from build123d import *

# Parameters (mm, degrees)
SKETCH_1_W          = 107
SKETCH_1_H          = 31
SKETCH_1_W_2        = 26
SKETCH_1_H_2        = 4
SKETCH_1_W_3        = 25
SKETCH_1_H_3        = 9
EXTRUDE_1_DEPTH     = 2
EXTRUDE_2_DEPTH     = 2
CUT_EXTRUDE_1_DEPTH = 117.228223767
SKETCH_5_W          = 15
SKETCH_5_H          = 2.5
EXTRUDE_3_DEPTH     = 2
CUT_EXTRUDE_2_DEPTH = 117.919844338
CUT_EXTRUDE_3_DEPTH = 117.919844338


with BuildPart() as part:
    # 草图1 → 凸台-拉伸1 (new body)
    with BuildSketch(Plane(origin=(0, 0, 0), x_dir=(0, 0, -1), z_dir=(1, 0, 0))):
        with Locations((53.5, 15.5)):
            Rectangle(SKETCH_1_W, SKETCH_1_H)
        with Locations((72, 16)):
            Rectangle(SKETCH_1_W_2, SKETCH_1_H_2, mode=Mode.SUBTRACT)
        with Locations((40.5, 18.5)):
            Rectangle(SKETCH_1_W_3, SKETCH_1_H_3, mode=Mode.SUBTRACT)
    extrude(amount=EXTRUDE_1_DEPTH)

    # 草图2 → 凸台-拉伸2 (add)
    with BuildSketch(Plane(origin=(2, 0, 0), x_dir=(0, 0, -1), z_dir=(1, 0, 0))):
        Polygon((0, 31), (-5, 31), (-5, 0), (0, 0), (0, 5), (-2.1, 5), (-2.1, 13), (0, 13), (0, 18), (-2.1, 18), (-2.1, 26), (0, 26), align=None)
        Polygon((107, 0), (107, 5), (109.1, 5), (109.1, 13), (107, 13), (107, 18), (109.1, 18), (109.1, 26), (107, 26), (107, 31), (112, 31), (112, 0), align=None)
    extrude(amount=-EXTRUDE_2_DEPTH)

    # 草图3 → 切除-拉伸1 (cut, through all)
    with BuildSketch(Plane(origin=(2, 0, 0), x_dir=(0, 0, -1), z_dir=(1, 0, 0))):
        with BuildLine():
            Line((-2.1, 24), (-2.1, 26))
            ThreePointArc((-2.1, 26), (-3.1, 25), (-2.1, 24))
        make_face()
        with BuildLine():
            Line((0, 24), (0, 26))
            ThreePointArc((0, 26), (1, 25), (0, 24))
        make_face()
        with BuildLine():
            Line((0, 20), (0, 18))
            ThreePointArc((0, 18), (1, 19), (0, 20))
        make_face()
        with BuildLine():
            Line((-2.1, 20), (-2.1, 18))
            ThreePointArc((-2.1, 18), (-3.1, 19), (-2.1, 20))
        make_face()
        with BuildLine():
            Line((-2.1, 11), (-2.1, 13))
            ThreePointArc((-2.1, 13), (-3.1, 12), (-2.1, 11))
        make_face()
        with BuildLine():
            Line((0, 11), (0, 13))
            ThreePointArc((0, 13), (1, 12), (0, 11))
        make_face()
        with BuildLine():
            Line((0, 7), (0, 5))
            ThreePointArc((0, 5), (1, 6), (0, 7))
        make_face()
        with BuildLine():
            Line((-2.1, 7), (-2.1, 5))
            ThreePointArc((-2.1, 5), (-3.1, 6), (-2.1, 7))
        make_face()
        with BuildLine():
            Line((109.1, 7), (109.1, 5))
            ThreePointArc((109.1, 5), (110.1, 6), (109.1, 7))
        make_face()
        with BuildLine():
            Line((107, 7), (107, 5))
            ThreePointArc((107, 5), (106, 6), (107, 7))
        make_face()
        with BuildLine():
            Line((107, 11), (107, 13))
            ThreePointArc((107, 13), (106, 12), (107, 11))
        make_face()
        with BuildLine():
            Line((109.1, 11), (109.1, 13))
            ThreePointArc((109.1, 13), (110.1, 12), (109.1, 11))
        make_face()
        with BuildLine():
            Line((109.1, 20), (109.1, 18))
            ThreePointArc((109.1, 18), (110.1, 19), (109.1, 20))
        make_face()
        with BuildLine():
            Line((107, 20), (107, 18))
            ThreePointArc((107, 18), (106, 19), (107, 20))
        make_face()
        with BuildLine():
            Line((107, 24), (107, 26))
            ThreePointArc((107, 26), (106, 25), (107, 24))
        make_face()
        with BuildLine():
            Line((109.1, 24), (109.1, 26))
            ThreePointArc((109.1, 26), (110.1, 25), (109.1, 24))
        make_face()
    extrude(amount=-CUT_EXTRUDE_1_DEPTH, mode=Mode.SUBTRACT)

    # 草图5 → 凸台-拉伸3 (add)
    with BuildSketch(Plane(origin=(2, 0, 0), x_dir=(0, 0, -1), z_dir=(1, 0, 0))):
        with Locations((17.5, 32.25)):
            Rectangle(SKETCH_5_W, SKETCH_5_H)
        with Locations((53.5, 32.25)):
            Rectangle(SKETCH_5_W, SKETCH_5_H)
        with Locations((89.5, 32.25)):
            Rectangle(SKETCH_5_W, SKETCH_5_H)
        with Locations((89.5, -1.25)):
            Rectangle(SKETCH_5_W, SKETCH_5_H)
        with Locations((53.5, -1.25)):
            Rectangle(SKETCH_5_W, SKETCH_5_H)
        with Locations((17.5, -1.25)):
            Rectangle(SKETCH_5_W, SKETCH_5_H)
    extrude(amount=-EXTRUDE_3_DEPTH)

    # 草图6 → 切除-拉伸2 (cut, through all)
    with BuildSketch(Plane(origin=(2, 0, 0), x_dir=(0, 0, -1), z_dir=(1, 0, 0))):
        with BuildLine():
            Line((10, 31), (8, 31))
            ThreePointArc((8, 31), (9, 30), (10, 31))
        make_face()
        with BuildLine():
            Line((25, 31), (27, 31))
            ThreePointArc((27, 31), (26, 30), (25, 31))
        make_face()
        with BuildLine():
            Line((46, 31), (44, 31))
            ThreePointArc((44, 31), (45, 30), (46, 31))
        make_face()
        with BuildLine():
            Line((61, 31), (63, 31))
            ThreePointArc((63, 31), (62, 30), (61, 31))
        make_face()
        with BuildLine():
            Line((82, 31), (80, 31))
            ThreePointArc((80, 31), (81, 30), (82, 31))
        make_face()
        with BuildLine():
            Line((97, 31), (99, 31))
            ThreePointArc((99, 31), (98, 30), (97, 31))
        make_face()
        with BuildLine():
            Line((97, 0), (99, 0))
            ThreePointArc((99, 0), (98, 1), (97, 0))
        make_face()
        with BuildLine():
            Line((82, 0), (80, 0))
            ThreePointArc((80, 0), (81, 1), (82, 0))
        make_face()
        with BuildLine():
            Line((61, 0), (63, 0))
            ThreePointArc((63, 0), (62, 1), (61, 0))
        make_face()
        with BuildLine():
            Line((46, 0), (44, 0))
            ThreePointArc((44, 0), (45, 1), (46, 0))
        make_face()
        with BuildLine():
            Line((25, 0), (27, 0))
            ThreePointArc((27, 0), (26, 1), (25, 0))
        make_face()
        with BuildLine():
            Line((10, 0), (8, 0))
            ThreePointArc((8, 0), (9, 1), (10, 0))
        make_face()
    extrude(amount=-CUT_EXTRUDE_2_DEPTH, mode=Mode.SUBTRACT)

    # 草图7 → 切除-拉伸3 (cut, through all)
    with BuildSketch(Plane(origin=(2, 0, 0), x_dir=(0, 0, -1), z_dir=(1, 0, 0))):
        with BuildLine():
            Line((6, 28), (22, 28))
            ThreePointArc((22, 28), (25, 25), (22, 22))
            Line((22, 22), (6, 22))
            ThreePointArc((6, 22), (3, 25), (6, 28))
        make_face()
        with BuildLine():
            Line((6, 10), (31, 10))
            ThreePointArc((31, 10), (34, 7), (31, 4))
            Line((31, 4), (6, 4))
            ThreePointArc((6, 4), (3, 7), (6, 10))
        make_face()
        with BuildLine():
            Line((6, 19), (22, 19))
            ThreePointArc((22, 19), (25, 16), (22, 13))
            Line((22, 13), (6, 13))
            ThreePointArc((6, 13), (3, 16), (6, 19))
        make_face()
        with BuildLine():
            Line((41, 10), (66, 10))
            ThreePointArc((66, 10), (69, 7), (66, 4))
            Line((66, 4), (41, 4))
            ThreePointArc((41, 4), (38, 7), (41, 10))
        make_face()
        with BuildLine():
            Line((76, 10), (101, 10))
            ThreePointArc((101, 10), (104, 7), (101, 4))
            Line((101, 4), (76, 4))
            ThreePointArc((76, 4), (73, 7), (76, 10))
        make_face()
        with BuildLine():
            Line((59, 28), (101, 28))
            ThreePointArc((101, 28), (104, 25), (101, 22))
            Line((101, 22), (59, 22))
            ThreePointArc((59, 22), (56, 25), (59, 28))
        make_face()
        with BuildLine():
            Line((91, 19), (101, 19))
            ThreePointArc((101, 19), (104, 16), (101, 13))
            Line((101, 13), (91, 13))
            ThreePointArc((91, 13), (88, 16), (91, 19))
        make_face()
    extrude(amount=-CUT_EXTRUDE_3_DEPTH, mode=Mode.SUBTRACT)


solid = part.part
Geometry check sheet. Reference: the model listing, model coordinates, mm. A direction names the side the tool comes from. Coordinates: 2 decimals unless noted, no trailing zeros. Order: outer loops, then holes, each group sorted by start corner. A loop starts at its lowest first (then second) coordinate and runs counter-clockwise, first axis right, second up. Notation, with made-up numbers: (18, -15) - (74, -15) arc R18 ccw to (74, 2) - close; hole circle Ø3 at (52.5, 36). An arc over 180 degrees is marked (long way). Answer in a Markdown table with one row per item. Add a question column.
1) Cross-section at D-D, the plane x = 1.2. State how many separate pieces and enclosed holes the cut face has, then the cut area to 3 significant figures.
2) Cross-section at B-B, the plane z = -9. Record the cut outline in (x, y), then the cut area to 3 significant figures.
3) Set-up check for faces 1 (the flat face through (1, 32, -25)), 2 (the flat face through (1, 31, -106)), 3 (the flat face through (1, 0, -71)), 4 (the cylindrical face through (1, 19, -106)): record each of +Z, -Z, +X, -X, +Y, -Y from which the full face is reachable in a straight line by a thin tool's end or side.
4) Cross-section at C-C, the plane z = -39. Record the cut outline in (x, y).
5) Release check for a two-part mould opening along Z. For faces 5 (the flat face through (1, 0, -35)), 6 (the flat face through (1, -2.5, -53)), 7 (the flat face through (1, 16, -112)) record: +Z half, -Z half, draft (parallel to the pull), parting line (faces both ways), or undercut.
6) Material ranges on line 1 along Y through (x, z) = (1.1, -45); line 2 along Y through (x, z) = (0.35, -76.5); line 3 along Y through (x, z) = (1.05, -17.5), recorded low to high. Write a range as [from, to].
7) Cross-section at A-A, the plane y = 25. Record the cut outline in (x, z).
8) Gauge pin test, flat ends, axial feed: P1, Ø0.6, axis at x = 1.5, z = -70, coming from the +Y side; P2, Ø0.6, axis at x = 1, y = 32, coming from the -Z side; P3, Ø0.6, axis at x = 1, z = -35.5, coming from the -Y side. Record the tip position at first contact, or that the pin passes through.
Check result:
| question | item | result |
|---|---|---|
| 1 | separate pieces | 1 |
| 1 | enclosed holes | 13 |
| 1 | area | 2,260 mm² |
| 2 | outline | (0, 1) - (2, 1) - (2, 4) - (0, 4) - close; (0, 10) - (2, 10) - (2, 13) - (0, 13) - close; (0, 19) - (2, 19) - (2, 22) - (0, 22) - close; (0, 28) - (2, 28) - (2, 30) - (0, 30) - close |
| 2 | area | 22.0 mm² |
| 3 | face 1 | +X, -X, +Y |
| 3 | face 2 | -Z, +X, -X, +Y |
| 3 | face 3 | +X, -X, -Y |
| 3 | face 4 | +X, -X |
| 4 | outline | (0, 0) - (2, 0) - (2, 4.76) - (0, 4.76) - close; (0, 9.24) - (2, 9.24) - (2, 14) - (0, 14) - close; (0, 23) - (2, 23) - (2, 31) - (0, 31) - close |
| 5 | face 5 | undercut |
| 5 | face 6 | draft |
| 5 | face 7 | -Z half |
| 6 | line 1 | y = [1, 4], [10, 14], [23, 30] |
| 6 | line 2 | y = [0, 4], [10, 14], [18, 22], [28, 31] |
| 6 | line 3 | y = [-2.5, 4], [10, 13], [19, 22], [28, 33.5] |
| 7 | outline | (0, -112) - (2, -112) - (2, -110.1) - (0, -110.1) - close; (0, -106) - (2, -106) - (2, -104) - (0, -104) - close; (0, -56) - (2, -56) - (2, -25) - (0, -25) - close; (0, -3) - (2, -3) - (2, -1) - (0, -1) - close; (0, 3.1) - (2, 3.1) - (2, 5) - (0, 5) - close |
| 8 | P1 | stops at y = 31 |
| 8 | P2 | stops at z = -97 |
| 8 | P3 | stops at y = 0 |
